Part print with two shaded views. Sizes in mm from the minimum x, y, z corner. Round coordinates to 2 decimals unless told otherwise and drop trailing zeros. Write each loop counter-clockwise with the first axis right and the second up, starting at its lowest first coordinate (ties: lowest second). Pieces come first, ordered by that corner, then holes.
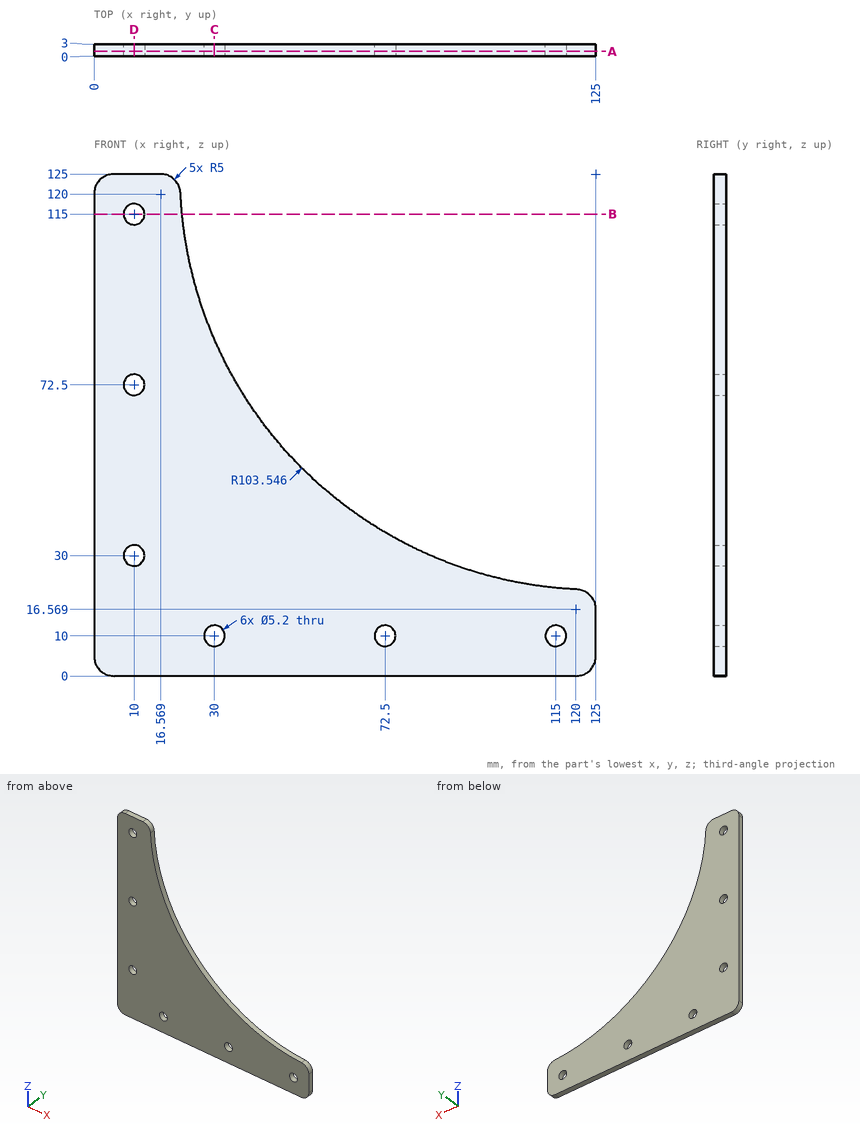
Q1. Cut at D-D on x = 10. Write the cut outline in (y, z), plus the area to 3 significant figures.
Values follow:
outline: (0, 0) - (3, 0) - (3, 27.4) - (0, 27.4) - close; (0, 32.6) - (3, 32.6) - (3, 69.9) - (0, 69.9) - close; (0, 75.1) - (3, 75.1) - (3, 112.4) - (0, 112.4) - close; (0, 117.6) - (3, 117.6) - (3, 125) - (0, 125) - close
area: 328 mm2
Q2. Cut at C-C on x = 30. Write the cut outline in (y, z), plus the area to 3 significant figures.
Values follow:
outline: (0, 0) - (3, 0) - (3, 7.4) - (0, 7.4) - close; (0, 12.6) - (3, 12.6) - (3, 83.81) - (0, 83.81) - close
area: 236 mm2
Q3. Cut at A-A on y = 1.15. Write the cut outline in (x, z).
Values follow:
outline: (0, 5) arc R5 ccw to (5, 0) - (120, 0) arc R5 ccw to (125, 5) - (125, 16.57) arc R5 ccw to (120.23, 21.56) arc R103.55 cw to (21.56, 120.23) arc R5 ccw to (16.57, 125) - (5, 125) arc R5 ccw to (0, 120) - close; hole circle Ø5.2 at (10, 30); hole circle Ø5.2 at (10, 72.5); hole circle Ø5.2 at (10, 115); hole circle Ø5.2 at (30, 10); hole circle Ø5.2 at (72.5, 10); hole circle Ø5.2 at (115, 10)
Q4. Cut at B-B on z = 115. Write the cut outline in (x, y).
Values follow:
outline: (0, 0) - (7.4, 0) - (7.4, 3) - (0, 3) - close; (12.6, 0) - (21.94, 0) - (21.94, 3) - (12.6, 3) - close
Q5. Wall check: L1, parallel to Z at x = 12, y = 0.2; L2, parallel to Z at x = 10, y = 1.65; L3, parallel to Z at x = 72.5, y = 2.35. Give the ranges that are in metal, low to high.
Values follow:
L1: z = 0 to 28.34, 31.66 to 70.84, 74.16 to 113.34, 116.66 to 125
L2: z = 0 to 27.4, 32.6 to 69.9, 75.1 to 112.4, 117.6 to 125
L3: z = 0 to 7.4, 12.6 to 35.75
Q6. Drop a flat-ended pin along its axis: pin 1 (1 mm diameter, centred on y = 2, z = 84.5, fed in from +X). Give the stop position or say it passes through.
Values follow:
pin 1: stops at x = 29.92
